from build123d import *

# Parameters (mm, degrees)
CUT_EXTRUDE1_DEPTH  = 5
SKETCH4_R           = 3.125
CUT_EXTRUDE2_DEPTH  = 3
CUT_EXTRUDE2_DRAFT  = -45
SKETCH12_R          = 3
BOSS_EXTRUDE1_DEPTH = 2.5


with BuildPart() as part:
    # Sketch2 → Revolve1 (revolve)
    with BuildSketch(Plane(origin=(0, 0, 0), x_dir=(0, 0, -1), z_dir=(1, 0, 0))):
        with BuildLine():
            Line((-10.5, 0), (-10.5, 4.7))
            Line((-10.5, 4.7), (-10.2, 5))
            Line((-10.2, 5), (-4.8, 5))
            Line((-4.8, 5), (-4.5, 4.7))
            Line((-4.5, 4.7), (-4.5, 3.3))
            ThreePointArc((-4.5, 3.3), (-4.412132034, 3.087867966), (-4.2, 3))
            Line((-4.2, 3), (9.850480947, 3))
            Line((9.850480947, 3), (10.5, 2.350480947))
            Line((10.5, 2.350480947), (10.5, 0))
            Line((10.5, 0), (-10.5, 0))
        make_face()
    revolve(axis=Axis((0, 0, -10.5), (0, 0, 1)))

    # Sketch3 → Cut-Extrude1 (cut)
    with BuildSketch(Plane.XY.offset(10.5)):
        Polygon((2.5, -1.443375673), (2.5, 1.443375673), (0, 2.886751346), (-2.5, 1.443375673), (-2.5, -1.443375673), (0, -2.886751346), align=None)
    extrude(amount=-CUT_EXTRUDE1_DEPTH, mode=Mode.SUBTRACT)


with BuildPart() as cut_extrude2_tool:
    # Sketch4 → Cut-Extrude2 (with draft: the straight prism first)
    with BuildSketch(Plane.XY.offset(10.5)):
        Circle(SKETCH4_R)
    extrude(amount=-CUT_EXTRUDE2_DEPTH)
    # Cut-Extrude2: the draft: its side faces are tilted about the plane it starts from
    cut_extrude2_sides = [cut_extrude2_tool.faces().sort_by_distance(p)[0] for p in [
        (-3.125, 0, 9),
    ]]
    draft(cut_extrude2_sides, Plane.XY.offset(10.5), CUT_EXTRUDE2_DRAFT)


with BuildPart() as part_1:
    add(part.part)

    # Cut-Extrude2: cut by cut_extrude2_tool
    add(cut_extrude2_tool.part, mode=Mode.SUBTRACT)


with BuildPart() as body_2:
    # Split1: the piece on the far side of the plane
    add(part_1.part)
    split(bisect_by=Plane.XY, keep=Keep.BOTTOM)


with BuildPart() as part_2:
    add(part_1.part)

    # Split1
    split(bisect_by=Plane.XY, keep=Keep.TOP)



with BuildPart() as body_2_1:
    # Body-Move/Copy1: moved
    add(body_2.part.moved(Location((0, 0, -2.5))))


with BuildPart() as part_3:
    add(part_2.part)

    add(body_2_1.part)  # Boss-Extrude1 merges body 2
    # Sketch12 → Boss-Extrude1 (add)
    with BuildSketch(Plane.XY.offset(-2.5)):
        with Locations(Location((0, 0, 0), (0, 0, 90))):
            Circle(SKETCH12_R)
    extrude(amount=BOSS_EXTRUDE1_DEPTH)


solid = part_3.part
Source: CAD feature listing. Evaluate the final solid. Frame: model axes, mm. A direction names the side the tool comes from. Give positions to 0.01 mm unless a question says otherwise; leave off trailing zeros. Order: outer loops, then holes, each group sorted by start corner. A loop starts at its lowest first (then second) coordinate and runs counter-clockwise, first axis right, second up. Notation, with made-up numbers: (56.25, -17.75) -> (76.25, -17.75) arc R26 cw to (76.25, 17.25) -> close; hole circle Ø7 at (58, 38.25). An arc over 180 degrees is marked (long way). Use a Markdown table: item, result.
1) Mould query, pull axis X, two halves, no side actions, for faces 4 (the flat face through (3, 2, 4.5)), 5 (the cylindrical face through (4.88, -1.08, 7.46)), 6 (the flat face through (1.233, -2.175, 7.914)), 7 (the flat face through (0, 0, 5.5)). Classes: +X half, -X half, draft (parallel to the pull), parting line (faces both ways), or undercut.
Answer list:
| item | result |
|---|---|
| face 4 | draft |
| face 5 | parting line |
| face 6 | undercut |
| face 7 | undercut |
2) Contact query for flat-ended pins moving along their axis: P1, Ø3, axis at x = -3.5, y = -3.5, coming from the +Z side; P2, Ø4, axis at x = -0.5, y = -0.5, coming from the +Z side; P3, Ø1.5, axis at x = 3.5, z = 3, coming from the +Y side; P4, Ø3, axis at y = -1.5, z = 2, coming from the -X side. Output: stop coordinate, or through.
Answer list:
| item | result |
|---|---|
| P1 | z = 10.5 |
| P2 | z = 10.08 |
| P3 | y = 1.2 |
| P4 | x = -3 |
3) Section query B-B, the plane z = 5.25. Return the cut outline in (x, y), then the cut area to 3 significant figures.
Answer list:
| item | result |
|---|---|
| outline | circle Ø10 at (0, 0) |
| area | 78.5 mm² |
4) Reachability of faces 1 (the flat face through (-1.267, -2.155, 7.914)), 2 (the flat face through (3.1, 1.1, 10.5)), 3 (the cylindrical face through (-0.9, 2.86, -4.19)) from +Z, -Z, +X, -X, +Y, -Y: full face, straight path, thin tool, end or side. Return the list, or none.
Answer list:
| item | result |
|---|---|
| face 1 | +Z |
| face 2 | +Z, +X, -X, +Y, -Y |
| face 3 | -Z |
5) Section query A-A, the plane y = 0. Return the cut outline in (x, z) (3 decimals), then the cut area to 3 significant figures.
Answer list:
| item | result |
|---|---|
| outline | (-5, 4.8) -> (-4.7, 4.5) -> (-3.3, 4.5) arc R0.3 cw to (-3, 4.2) -> (-3, -12.35) -> (-2.35, -13) -> (2.35, -13) -> (3, -12.35) -> (3, 4.2) arc R0.3 cw to (3.3, 4.5) -> (4.7, 4.5) -> (5, 4.8) -> (5, 10.2) -> (4.7, 10.5) -> (3.125, 10.5) -> (2.5, 9.875) -> (2.5, 5.5) -> (-2.5, 5.5) -> (-2.5, 9.875) -> (-3.125, 10.5) -> (-4.7, 10.5) -> (-5, 10.2) -> close |
| area | 139 mm² |
6) Ray query, line 1 along Z through (x, y) = (-1.75, 0); line 2 along Z through (x, y) = (4.5, 1); line 3 along X through (y, z) = (2, 2.25). Return the intervals inside material, ascending. Write a range as [from, to].
Answer list:
| item | result |
|---|---|
| line 1 | [-13, 5.5] |
| line 2 | [4.5, 10.5] |
| line 3 | [-2.24, 2.24] |
7) Section query C-C, the plane z = -6.25. Return the cut outline in (x, y).
Answer list:
| item | result |
|---|---|
| outline | circle Ø6 at (0, 0) |
